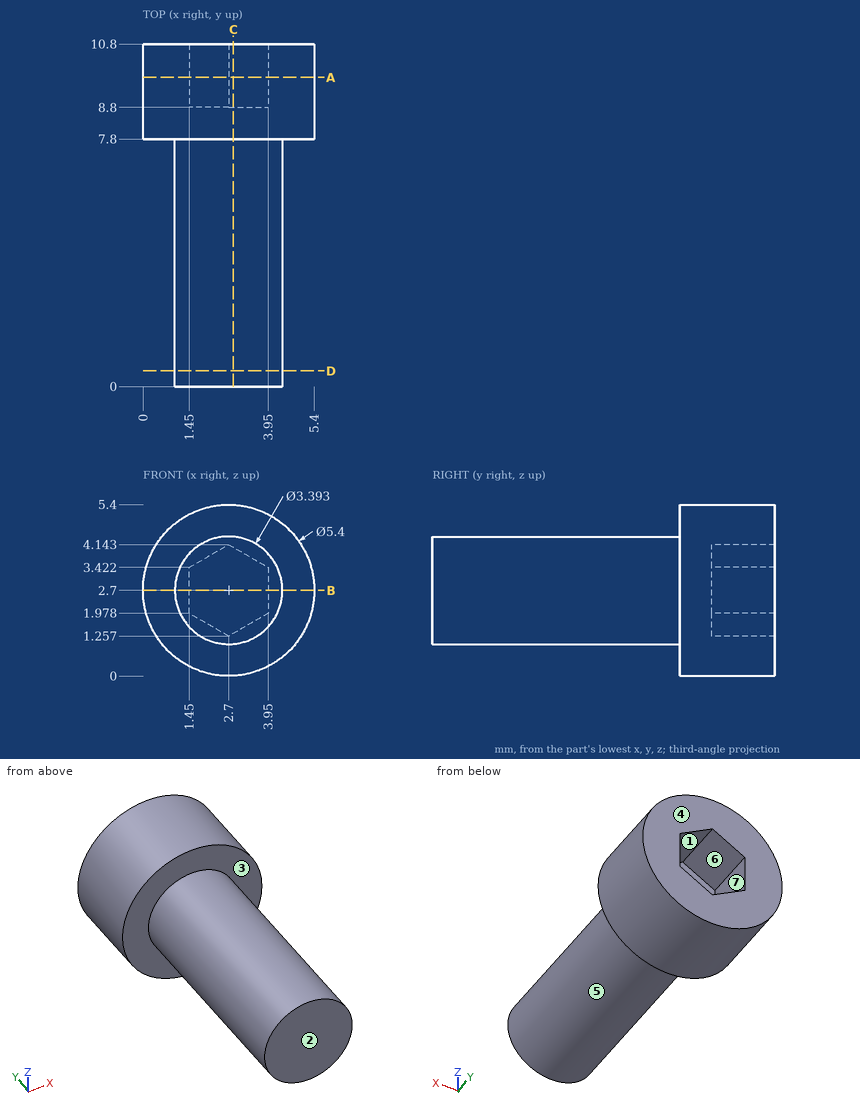
Design review of the part shown in the three views and the two pictorial views. Dimensions are in mm from the part's minimum x, y and z. A direction names the side the tool comes from. Give positions to 0.01 mm unless a question says otherwise; leave off trailing zeros. Loops run counter-clockwise (first coordinate to the right, second up) from the corner with the lowest first, then second, coordinate; pieces in that order, holes last. Notation, with made-up numbers: (22.5, 79) -> (79.5, 79) arc R19 cw to (79.5, 97) -> close; hole circle Ø1 at (53.25, 36). An arc over 180 degrees is marked (long way). Write each question's results on one line, items separated by ' | '.
Q1. Take a section at A-A, the plane y = 9.75. Write out the cut boundary in (x, z).
Reply:
outline: circle Ø5.4 at (2.7, 2.7); hole (1.45, 1.98) -> (2.7, 1.26) -> (3.95, 1.98) -> (3.95, 3.42) -> (2.7, 4.14) -> (1.45, 3.42) -> close
Q2. Take a section at B-B, the plane z = 2.7. Write out the cut boundary in (x, y).
Reply:
outline: (0, 7.8) -> (1, 7.8) -> (1, 0) -> (4.4, 0) -> (4.4, 7.8) -> (5.4, 7.8) -> (5.4, 10.8) -> (3.95, 10.8) -> (3.95, 8.8) -> (1.45, 8.8) -> (1.45, 10.8) -> (0, 10.8) -> close
Q3. Machinability: for the marked faces 1, 2 and 3, which of the approach directions +Z, -Z, +X, -X, +Y, -Y give a long, thin tool a straight path to every point of the face, cutting with its end or side? Answer none if there is none.
Reply:
face 1: +Y | face 2: +Z, -Z, +X, -X, -Y | face 3: -Y
Q4. The part is to be moulded in two halves that separate along X. For the marked faces 4, 5, 6 and 7, say which applies: +X half, -X half, draft (parallel to the pull), parting line (faces both ways), or undercut.
Reply:
face 4: draft | face 5: parting line | face 6: undercut | face 7: undercut
Q5. Wall thickness on L1, parallel to Y at x = 5, z = 3; L2, parallel to Y at x = 1.55, z = 3.3; L3, parallel to Z at x = 4, y = 3.5: over which ranges is each line inside the solid? List them lowest first.
Reply:
L1: y = 7.8 to 10.8 | L2: y = 0 to 8.8 | L3: z = 1.61 to 3.79
Q6. For pin 1 Ø0.8 at (x, z) = (3, 3) entering from +Y; pin 2 Ø1 at (x, y) = (4, 2.5) entering from +Z (1 decimal); pin 3 Ø1.5 at (y, z) = (9.5, 1.5) entering from -X, all flat-tipped, find the tip position at first contact; note any pin that passes through.
Reply:
pin 1: stops at y = 8.8 | pin 2: stops at z = 4.2 | pin 3: stops at x = 0.04
Q7. Take a section at D-D, the plane y = 0.5. Write out the cut boundary in (x, z).
Reply:
outline: circle Ø3.39 at (2.7, 2.7)
Q8. Take a section at C-C, the plane x = 2.85. Write out the cut boundary in (y, z) (1 decimal), plus the area to 3 significant figures.
Reply:
outline: (0, 1) -> (7.8, 1) -> (7.8, 0) -> (10.8, 0) -> (10.8, 1.3) -> (8.8, 1.3) -> (8.8, 4.1) -> (10.8, 4.1) -> (10.8, 5.4) -> (7.8, 5.4) -> (7.8, 4.4) -> (0, 4.4) -> close | area: 37.1 mm²
